For this review, take the finished solid that the model builds, in its own axes (mm). Face numbers are marked on the shaded views. A direction names the side the tool comes from. Coordinates: 2 decimals unless noted, no trailing zeros. Write each loop counter-clockwise with the first axis right and the second up, starting at its lowest first coordinate (ties: lowest second). Pieces come first, ordered by that corner, then holes. Notation, with made-up numbers: M 17.5,85.25 L 57.5,85.25 A9 cw 57.5,92.25 Z; hole C 43.25,76 d8. An arc over 180 degrees is marked long. One line per question, with ' | ' between items.
from build123d import *

# Parameters (mm, degrees)
SKETCH1_W           = 127
SKETCH1_H           = 76.2
BOSS_EXTRUDE1_DEPTH = 76.2
SKETCH2_R           = 19.05
BOSS_EXTRUDE2_DEPTH = 5.08
SKETCH3_R           = 1.27
BOSS_EXTRUDE3_DEPTH = 152.4


with BuildPart() as part:
    # Sketch1 → Boss-Extrude1 (new body)
    with BuildSketch(Plane.XY):
        Rectangle(SKETCH1_W, SKETCH1_H)
    extrude(amount=BOSS_EXTRUDE1_DEPTH)

    # Sketch2 → Boss-Extrude2 (add)
    with BuildSketch(Plane.XY.offset(76.2)):
        with Locations((38.1, 0)):
            Circle(SKETCH2_R)
        with Locations((-38.1, 0)):
            Circle(SKETCH2_R)
    extrude(amount=BOSS_EXTRUDE2_DEPTH)

    # Sketch3 → Boss-Extrude3 (add)
    with BuildSketch(Plane.XY.offset(81.28)):
        with Locations(Location((41.35063463, -3.592102448, 0), (0, 0, 180))):
            Circle(SKETCH3_R)
        with Locations(Location((34.166429733, 3.592102448, 0), (0, 0, 180))):
            Circle(SKETCH3_R)
        with Locations(Location((-41.755190332, -3.592102448, 0), (0, 0, 180))):
            Circle(SKETCH3_R)
        with Locations(Location((-34.570985435, 3.592102448, 0), (0, 0, 180))):
            Circle(SKETCH3_R)
    extrude(amount=BOSS_EXTRUDE3_DEPTH)


solid = part.part
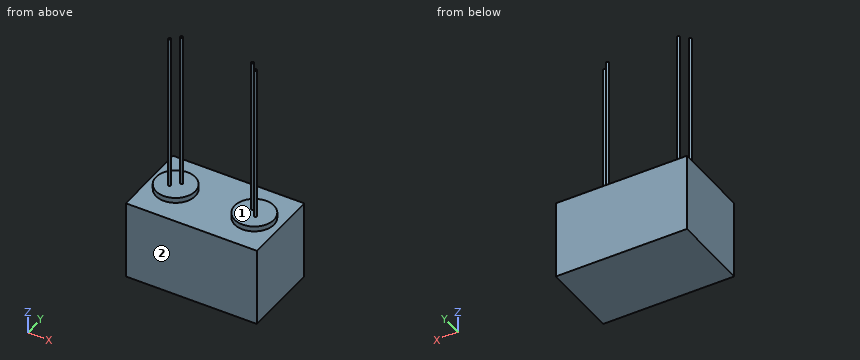
1) Machinability: for the marked faces 1 and 2, which of the approach directions +Z, -Z, +X, -X, +Y, -Y give a long, thin tool a straight path to every point of the face, cutting with its end or side? Answer none if there is none.
Responses:
face 1: +Z | face 2: +Z, -Z, +X, -X, -Y
2) Insertion check: pin 1 Ø12 at (x, y) = (-41, 25) entering from +Z. The pin has a flat end and moves straight along its axis. Give the tip position at first contact, or say it passes through.
Responses:
pin 1: z = 76.2
3) We need section C-C on z = 212.5. State the section outline as (x, y) points, then the cut area to 3 significant figures.
Responses:
outline: C -41.76,-3.59 d2.54; C -34.57,3.59 d2.54; C 34.17,3.59 d2.54; C 41.35,-3.59 d2.54 | area: 20.3 mm^2
4) To check wall thickness, follow line 1 along Z through (x, y) = (47, 21); line 2 along Z through (x, y) = (-35.5, 16); line 3 along Y through (x, z) = (-34.5, 134.5). State the ranges of each line that lie inside material, in increasing order. Write a range as [from, to].
Responses:
line 1: [0, 76.2] | line 2: [0, 81.28] | line 3: [2.32, 4.86]
5) We need section A-A on y = 0. State the section outline as (x, z) points, then the cut area to 3 significant figures.
Responses:
outline: M -63.5,0 L 63.5,0 L 63.5,76.2 L 57.15,76.2 L 57.15,81.28 L 19.05,81.28 L 19.05,76.2 L -19.05,76.2 L -19.05,81.28 L -57.15,81.28 L -57.15,76.2 L -63.5,76.2 Z | area: 10,100 mm^2
6) We need section B-B on x = -38.1. State the section outline as (y, z) points.
Responses:
outline: M -38.1,0 L 38.1,0 L 38.1,76.2 L 19.05,76.2 L 19.05,81.28 L -19.05,81.28 L -19.05,76.2 L -38.1,76.2 Z
7) We need section D-D on y = -30.5. State the section outline as (x, z) points.
Responses:
outline: M -63.5,0 L 63.5,0 L 63.5,76.2 L -63.5,76.2 Z
